Part model, mm, in its own coordinate system. A direction names the side the tool comes from. Round coordinates to 2 decimals unless told otherwise and drop trailing zeros. Write each loop counter-clockwise with the first axis right and the second up, starting at its lowest first coordinate (ties: lowest second). Pieces come first, ordered by that corner, then holes. Notation, with made-up numbers: M 70,13 L 102,13 A17 ccw 102,41 Z; hole C -6,30.5 d3. An arc over 180 degrees is marked long. Answer as a JSON object with one key per item and string values. Group by question number.
1. Drill centre lines: line 1 (X direction, y = -8.4, z = 0); line 2 (X direction, y = -6.5, z = 1.75); line 3 (Y direction, x = -4, z = -0.5). Where is each one in solid material? Low to high. Write a range as from..to.
2. Band-saw the part on B-B, the plane z = 0. Write the cut outline in (x, y), plus the area to 3 significant figures.
3. Band-saw the part on A-A, the plane x = -5. Write the cut outline in (y, z), plus the area to 3 significant figures.
4. Two-plate mould, pull along X, no slides. Class faces 1 (the face through (-16, -6, 0)), 2 (the face through (0, -11, 0)), 3 (the face through (-5, -6, 0)), 4 (the face through (-21, 0, 0)): +X half, -X half, draft (parallel to the pull), parting line (faces both ways), or undercut.
5. Band-saw the part on C-C, the plane y = -8. Write the cut outline in (x, z), plus the area to 3 significant figures.
6. Which spindle directions (+Z, -Z, +X, -X, +Y, -Y) get a long thin tool onto all of the face, cutting with end or side? Do faces 5 (the face through (0, 0, 5)), 6 (the face through (-14, -9, 0)). Say none if no direction does.
7. Drop a flat-ended pin along its axis: pin 1 (1.2 mm diameter, centred on x = -16, z = 1, fed in from -Y). Give the stop position or say it passes through.
from build123d import *

# Parameters (mm, degrees)
SKETCH2_W           = 10
SKETCH2_H           = 22
BOSS_EXTRUDE1_DEPTH = 21
SKETCH3_R           = 2
CUT_EXTRUDE1_DEPTH  = 5


with BuildPart() as part:
    # Sketch2 → Boss-Extrude1 (new, symmetric)
    with BuildSketch(Plane(origin=(0, 0, 0), x_dir=(0, 0, -1), z_dir=(1, 0, 0))):
        Rectangle(SKETCH2_W, SKETCH2_H)
    extrude(amount=BOSS_EXTRUDE1_DEPTH, both=True)

    # Sketch3 → Cut-Extrude1 (cut)
    with BuildSketch(Plane.XZ.offset(11)):
        with Locations(Location((-16, 0, 0), (0, 0, 270))):
            Circle(SKETCH3_R)
        with Locations(Location((-5, 0, 0), (0, 0, 270))):
            Circle(SKETCH3_R)
    extrude(amount=-CUT_EXTRUDE1_DEPTH, mode=Mode.SUBTRACT)


solid = part.part
Worked answers:
{
 "1": {"line 1": "x = -21..-18, -14..-7, -3..21", "line 2": "x = -21..-16.97, -15.03..-5.97, -4.03..21", "line 3": "y = -6..11"},
 "2": {"outline": "M -21,-11 L -18,-11 L -18,-6 L -14,-6 L -14,-11 L -7,-11 L -7,-6 L -3,-6 L -3,-11 L 21,-11 L 21,11 L -21,11 Z", "area": "884 mm^2"},
 "3": {"outline": "M -11,-5 L 11,-5 L 11,5 L -11,5 L -11,2 L -6,2 L -6,-2 L -11,-2 Z", "area": "200 mm^2"},
 "4": {"face 1": "undercut", "face 2": "draft", "face 3": "undercut", "face 4": "-X half"},
 "5": {"outline": "M -21,-5 L 21,-5 L 21,5 L -21,5 Z; hole C -16,0 d4; hole C -5,0 d4", "area": "395 mm^2"},
 "6": {"face 5": "+Z, +X, -X, +Y, -Y", "face 6": "-Y"},
 "7": {"pin 1": "stops at y = -6"}
}
